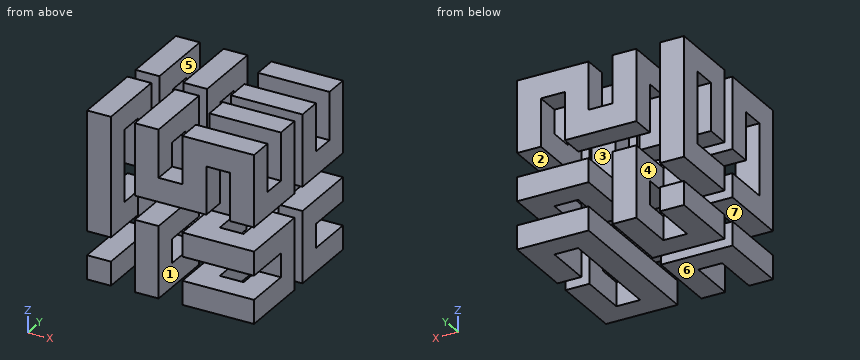
```python
from build123d import *

# Parameters (mm, degrees)
F0_W      = 6.35
F0_H      = 6.35
F1_DEPTH  = 19.05
F2_W      = 6.35
F2_H      = 6.35
F3_DEPTH  = 19.05
F4_W      = 6.35
F4_H      = 6.35
F5_DEPTH  = 19.05
F6_W      = 6.35
F6_H      = 6.35
F7_DEPTH  = 19.05
F8_W      = 6.35
F8_H      = 6.35
F9_DEPTH  = 19.05
F10_W     = 6.35
F10_H     = 6.35
F11_DEPTH = 19.05
F12_W     = 6.35
F12_H     = 6.35
F13_DEPTH = 19.05
F14_W     = 6.35
F14_H     = 6.35
F15_DEPTH = 31.75
F16_W     = 6.35
F16_H     = 6.35
F17_DEPTH = 19.05
F18_W     = 6.35
F18_H     = 6.35
F19_DEPTH = 19.05
F20_W     = 6.35
F20_H     = 6.35
F21_DEPTH = 19.05
F22_W     = 6.35
F22_H     = 6.35
F23_DEPTH = 19.05
F24_W     = 6.35
F24_H     = 6.35
F25_DEPTH = 19.05
F26_W     = 6.35
F26_H     = 6.35
F27_DEPTH = 19.05
F28_W     = 6.35
F28_H     = 6.35
F29_DEPTH = 19.05
F30_W     = 6.35
F30_H     = 6.35
F31_DEPTH = 19.05
F32_W     = 6.35
F32_H     = 6.35
F33_DEPTH = 19.05
F34_W     = 6.35
F34_H     = 6.35
F35_DEPTH = 19.05
F36_W     = 6.35
F36_H     = 6.35
F37_DEPTH = 19.05
F38_W     = 6.35
F38_H     = 6.35
F39_DEPTH = 19.05
F40_W     = 6.35
F40_H     = 6.35
F41_DEPTH = 19.05
F42_W     = 6.35
F42_H     = 6.35
F43_DEPTH = 31.75
F44_W     = 6.35
F44_H     = 6.35
F45_DEPTH = 19.05
F46_W     = 6.35
F46_H     = 6.35
F47_DEPTH = 19.05
F48_W     = 6.35
F48_H     = 6.35
F49_DEPTH = 19.05
F50_W     = 6.35
F50_H     = 6.35
F51_DEPTH = 19.05
F52_W     = 6.35
F52_H     = 6.35
F53_DEPTH = 19.05
F54_W     = 6.35
F54_H     = 6.35
F55_DEPTH = 19.05
F56_W     = 6.35
F56_H     = 6.35
F57_DEPTH = 20.955


with BuildPart() as f1:
    # F0 (on Front) → F1 (new body)
    with BuildSketch(Plane.XZ):
        with Locations((3.175, 3.175)):
            Rectangle(F0_W, F0_H)
    extrude(amount=F1_DEPTH)

    # F2 (on face) → F3 (join)
    with BuildSketch(Plane(origin=(0, 0, 0), x_dir=(0, -1, 0), z_dir=(-1, 0, 0))):
        with Locations((15.875, 3.175)):
            Rectangle(F2_W, F2_H)
    extrude(amount=-F3_DEPTH)

    # F4 (on face) → F5 (join)
    with BuildSketch(Plane.XZ.offset(19.05)):
        with Locations((15.875, 3.175)):
            Rectangle(F4_W, F4_H)
    extrude(amount=-F5_DEPTH)

    # F6 (on face) → F7 (join)
    with BuildSketch(Plane(origin=(0, 0, 0), x_dir=(1, 0, 0), z_dir=(0, 0, -1))):
        with Locations((15.875, 3.175)):
            Rectangle(F6_W, F6_H)
    extrude(amount=-F7_DEPTH)

    # F8 (on face) → F9 (join)
    with BuildSketch(Plane(origin=(0, 0, 0), x_dir=(-1, 0, 0), z_dir=(0, 1, 0))):
        with Locations((-15.875, 15.875)):
            Rectangle(F8_W, F8_H)
    extrude(amount=-F9_DEPTH)

    # F10 (on face) → F11 (join)
    with BuildSketch(Plane.YZ.offset(19.05)):
        with Locations((-15.875, 15.875)):
            Rectangle(F10_W, F10_H)
    extrude(amount=-F11_DEPTH)

    # F12 (on face) → F13 (join)
    with BuildSketch(Plane.XZ.offset(19.05)):
        with Locations((3.175, 15.875)):
            Rectangle(F12_W, F12_H)
    extrude(amount=-F13_DEPTH)

    # F14 (on face) → F15 (join)
    with BuildSketch(Plane(origin=(0, 0, 12.7), x_dir=(1, 0, 0), z_dir=(0, 0, -1))):
        with Locations((3.175, 3.175)):
            Rectangle(F14_W, F14_H)
    extrude(amount=-F15_DEPTH)

    # F16 (on face) → F17 (join)
    with BuildSketch(Plane(origin=(0, 0, 0), x_dir=(-1, 0, 0), z_dir=(0, 1, 0))):
        with Locations((-3.175, 41.275)):
            Rectangle(F16_W, F16_H)
    extrude(amount=-F17_DEPTH)

    # F18 (on face) → F19 (join)
    with BuildSketch(Plane.XY.offset(44.45)):
        with Locations((3.175, -15.875)):
            Rectangle(F18_W, F18_H)
    extrude(amount=-F19_DEPTH)

    # F20 (on face) → F21 (join)
    with BuildSketch(Plane(origin=(0, 0, 0), x_dir=(0, -1, 0), z_dir=(-1, 0, 0))):
        with Locations((15.875, 28.575)):
            Rectangle(F20_W, F20_H)
    extrude(amount=-F21_DEPTH)

    # F22 (on face) → F23 (join)
    with BuildSketch(Plane(origin=(0, 0, 25.4), x_dir=(1, 0, 0), z_dir=(0, 0, -1))):
        with Locations((15.875, 15.875)):
            Rectangle(F22_W, F22_H)
    extrude(amount=-F23_DEPTH)

    # F24 (on face) → F25 (join)
    with BuildSketch(Plane.XZ.offset(19.05)):
        with Locations((15.875, 41.275)):
            Rectangle(F24_W, F24_H)
    extrude(amount=-F25_DEPTH)

    # F26 (on face) → F27 (join)
    with BuildSketch(Plane.XY.offset(44.45)):
        with Locations((15.875, -3.175)):
            Rectangle(F26_W, F26_H)
    extrude(amount=-F27_DEPTH)

    # F28 (on face) → F29 (join)
    with BuildSketch(Plane(origin=(12.7, 0, 0), x_dir=(0, -1, 0), z_dir=(-1, 0, 0))):
        with Locations((3.175, 28.575)):
            Rectangle(F28_W, F28_H)
    extrude(amount=-F29_DEPTH)

    # F30 (on face) → F31 (join)
    with BuildSketch(Plane(origin=(0, 0, 25.4), x_dir=(1, 0, 0), z_dir=(0, 0, -1))):
        with Locations((28.575, 3.175)):
            Rectangle(F30_W, F30_H)
    extrude(amount=-F31_DEPTH)

    # F32 (on face) → F33 (join)
    with BuildSketch(Plane(origin=(25.4, 0, 0), x_dir=(0, -1, 0), z_dir=(-1, 0, 0))):
        with Locations((3.175, 41.275)):
            Rectangle(F32_W, F32_H)
    extrude(amount=-F33_DEPTH)

    # F34 (on face) → F35 (join)
    with BuildSketch(Plane.XY.offset(44.45)):
        with Locations((41.275, -3.175)):
            Rectangle(F34_W, F34_H)
    extrude(amount=-F35_DEPTH)

    # F36 (on face) → F37 (join)
    with BuildSketch(Plane(origin=(0, 0, 0), x_dir=(-1, 0, 0), z_dir=(0, 1, 0))):
        with Locations((-41.275, 28.575)):
            Rectangle(F36_W, F36_H)
    extrude(amount=-F37_DEPTH)

    # F38 (on face) → F39 (join)
    with BuildSketch(Plane(origin=(0, 0, 25.4), x_dir=(1, 0, 0), z_dir=(0, 0, -1))):
        with Locations((41.275, 15.875)):
            Rectangle(F38_W, F38_H)
    extrude(amount=-F39_DEPTH)

    # F40 (on face) → F41 (join)
    with BuildSketch(Plane.YZ.offset(44.45)):
        with Locations((-15.875, 41.275)):
            Rectangle(F40_W, F40_H)
    extrude(amount=-F41_DEPTH)

    # F42 (on face) → F43 (join)
    with BuildSketch(Plane.XY.offset(44.45)):
        with Locations((28.575, -15.875)):
            Rectangle(F42_W, F42_H)
    extrude(amount=-F43_DEPTH)

    # F44 (on face) → F45 (join)
    with BuildSketch(Plane.XZ.offset(19.05)):
        with Locations((28.575, 15.875)):
            Rectangle(F44_W, F44_H)
    extrude(amount=-F45_DEPTH)

    # F46 (on face) → F47 (join)
    with BuildSketch(Plane(origin=(25.4, 0, 0), x_dir=(0, -1, 0), z_dir=(-1, 0, 0))):
        with Locations((3.175, 15.875)):
            Rectangle(F46_W, F46_H)
    extrude(amount=-F47_DEPTH)

    # F48 (on face) → F49 (join)
    with BuildSketch(Plane(origin=(0, 0, 0), x_dir=(-1, 0, 0), z_dir=(0, 1, 0))):
        with Locations((-41.275, 15.875)):
            Rectangle(F48_W, F48_H)
    extrude(amount=-F49_DEPTH)

    # F50 (on face) → F51 (join)
    with BuildSketch(Plane.XY.offset(19.05)):
        with Locations((41.275, -15.875)):
            Rectangle(F50_W, F50_H)
    extrude(amount=-F51_DEPTH)

    # F52 (on face) → F53 (join)
    with BuildSketch(Plane.XZ.offset(19.05)):
        with Locations((41.275, 3.175)):
            Rectangle(F52_W, F52_H)
    extrude(amount=-F53_DEPTH)

    # F54 (on face) → F55 (join)
    with BuildSketch(Plane.YZ.offset(44.45)):
        with Locations((-3.175, 3.175)):
            Rectangle(F54_W, F54_H)
    extrude(amount=-F55_DEPTH)

    # F56 (on face) → F57 (join)
    with BuildSketch(Plane(origin=(0, 0, 0), x_dir=(-1, 0, 0), z_dir=(0, 1, 0))):
        with Locations((-28.575, 3.175)):
            Rectangle(F56_W, F56_H)
    extrude(amount=-F57_DEPTH)

    # F58: F1 across face


with BuildPart() as f1_1:
    add(f1.part)
    add(f1.part.mirror(Plane(origin=(28.575, -20.955, 3.175), x_dir=(-1, 0, 0), z_dir=(0, -1, 0))))


solid = f1_1.part
```
Could you check a few things on this model? Use its own coordinates, in mm. Face numbers are marked on the shaded views. A direction names the side the tool comes from. Coordinates: 2 decimals unless noted, no trailing zeros. Write each loop counter-clockwise with the first axis right and the second up, starting at its lowest first coordinate (ties: lowest second). Pieces come first, ordered by that corner, then holes. Notation, with made-up numbers: (-40, 37) -> (-13, 37) arc R31 cw to (-13, 72) -> close; hole circle Ø5 at (58, 74). An arc over 180 degrees is marked (long way). One line per question, with ' | ' between items. Start each with the question number.
1. Please list where these lines run through material, in increasing order: line 1 along Y through (x, z) = (37.5, 40); line 2 along Z through (x, y) = (42, -11.5).
2. If we section it at C-C (x = 22): Please give me the cut outline in (y, z).
3. Thinking about a two-plate mould opening in Z: for the marked faces 5, 6 and 7, which applies, pulls with the +Z half, pulls with the -Z half, needs draft (parallel to the pull), parting line crosses it, or undercut?
4. Will these pins go through, and if not, where does the flat tip stop? P1, Ø1.9, axis at x = 8, z = 2.5, coming from the -Y side; P2, Ø5, axis at x = 22, y = -3.5, coming from the +Z side.
5. If we section it at A-A (y = -24): Count the separate pieces of the cut face and the enclosed holes in it, and give its area (3 significant figures).
6. For the marked faces 1, 2, 3 and 4, which set-ups out of +Z, -Z, +X, -X, +Y, -Y let a thin tool reach every point of the face, with its end or its side?
Return value:
1) line 1: y = -41.91 to -35.56, -29.21 to -22.86, -19.05 to -12.7, -6.35 to 0 | line 2: z = 0 to 6.35, 12.7 to 19.05, 25.4 to 31.75
2) outline: (-41.91, 25.4) -> (-35.56, 25.4) -> (-35.56, 31.75) -> (-41.91, 31.75) -> close; (-6.35, 25.4) -> (0, 25.4) -> (0, 31.75) -> (-6.35, 31.75) -> close
3) face 5: needs draft | face 6: pulls with the -Z half | face 7: undercut
4) P1: stops at y = -29.21 | P2: stops at z = 31.75
5) separate pieces: 6 | enclosed holes: 0 | area: 1,050 mm²
6) face 1: -Z, +Y, -Y | face 2: +X, +Y, -Y | face 3: +Z | face 4: +Z, -Z, +Y
